Could you check a few things on this model? Use its own coordinates, in mm. A direction names the side the tool comes from. Coordinates: 2 decimals unless noted, no trailing zeros. Loops run counter-clockwise (first coordinate to the right, second up) from the corner with the lowest first, then second, coordinate; pieces in that order, holes last. Notation, with made-up numbers: M 22,-31 L 67,-31 A13 cw 67,-24 Z; hole C -39.5,-26.75 d4. An arc over 180 degrees is marked long. Use one line per item in the form item = value. Start each with the question number.
```python
from build123d import *

# Parameters (mm, degrees)
SKETCH2_R          = 17.5
CUT_EXTRUDE1_DEPTH = 108.121426428
SKETCH3_W          = 10
SKETCH3_H          = 6.6
CUT_EXTRUDE2_DEPTH = 108.121426428
SKETCH4_R          = 4
CUT_EXTRUDE3_DEPTH = 10
CUT_EXTRUDE4_DEPTH = 108.121426428


with BuildPart() as part:
    # Sketch1 → Revolve1 (revolve)
    with BuildSketch(Plane.XY, mode=Mode.PRIVATE) as revolve1_sk:
        with BuildLine():
            Line((-55, 0), (0, 0))
            Line((0, 0), (0, 65))
            Line((0, 65), (-15, 65))
            ThreePointArc((-15, 65), (-18.535533906, 63.535533906), (-20, 60))
            Line((-20, 60), (-20, 38))
            ThreePointArc((-20, 38), (-22.343145751, 32.343145751), (-28, 30))
            Line((-28, 30), (-52, 30))
            ThreePointArc((-52, 30), (-54.121320344, 29.121320344), (-55, 27))
            Line((-55, 27), (-55, 0))
        make_face()
    revolve(revolve1_sk.sketch.rotate(Axis((-55, 0, 0), (1, 0, 0)), 90), axis=Axis((-55, 0, 0), (1, 0, 0)))

    # Sketch2 → Cut-Extrude1 (cut, through all)
    with BuildSketch(Plane.ZY.offset(55)):
        Circle(SKETCH2_R)
    extrude(amount=-CUT_EXTRUDE1_DEPTH, mode=Mode.SUBTRACT)

    # Sketch3 → Cut-Extrude2 (cut, through all)
    with BuildSketch(Plane(origin=(0, 0, 0), x_dir=(0, 0, -1), z_dir=(1, 0, 0))):
        with Locations((0, 17.5)):
            Rectangle(SKETCH3_W, SKETCH3_H)
    extrude(amount=-CUT_EXTRUDE2_DEPTH, mode=Mode.SUBTRACT)

    # Sketch4 → Cut-Extrude3 (cut)
    with BuildSketch(Plane(origin=(0, -30, 0), x_dir=(-1, 0, 0), z_dir=(0, -1, 0))):
        with Locations(Location((40.229772479, 0, 0), (0, 0, 90))):
            Circle(SKETCH4_R)
    extrude(amount=-CUT_EXTRUDE3_DEPTH, mode=Mode.SUBTRACT)

    # Sketch5 → Cut-Extrude4 (cut, through all)
    with BuildSketch(Plane(origin=(0, 0, 0), x_dir=(0, 0, -1), z_dir=(1, 0, 0))):
        with BuildLine():
            ThreePointArc((-48.88940991, 26.321058084), (-49.547284726, 19.781093542), (-45.084090379, 14.955761253))
            ThreePointArc((-45.084090379, 14.955761253), (-41.13620668, 23.75), (-35.494114368, 31.566086948))
            ThreePointArc((-35.494114368, 31.566086948), (-41.904571885, 33.01866049), (-47.23940991, 29.178941916))
            Line((-47.23940991, 29.178941916), (-48.88940991, 26.321058084))
        make_face()
        with BuildLine():
            ThreePointArc((-35.494114368, 31.566086948), (-41.13620668, 23.75), (-45.084090379, 14.955761253))
            ThreePointArc((-45.084090379, 14.955761253), (-39.421242138, 14.734980037), (-35.033003449, 18.321058084))
            Line((-35.033003449, 18.321058084), (-33.383003449, 21.178941916))
            ThreePointArc((-33.383003449, 21.178941916), (-32.471488106, 26.772307122), (-35.494114368, 31.566086948))
        make_face()
        with BuildLine():
            ThreePointArc((35.033003449, 18.321058084), (39.421242138, 14.734980037), (45.084090379, 14.955761253))
            ThreePointArc((45.084090379, 14.955761253), (41.13620668, 23.75), (35.494114368, 31.566086948))
            ThreePointArc((35.494114368, 31.566086948), (32.471488106, 26.772307122), (33.383003449, 21.178941916))
            Line((33.383003449, 21.178941916), (35.033003449, 18.321058084))
        make_face()
        with BuildLine():
            ThreePointArc((35.494114368, 31.566086948), (41.13620668, 23.75), (45.084090379, 14.955761253))
            ThreePointArc((45.084090379, 14.955761253), (49.547284726, 19.781093542), (48.88940991, 26.321058084))
            Line((48.88940991, 26.321058084), (47.23940991, 29.178941916))
            ThreePointArc((47.23940991, 29.178941916), (41.904571885, 33.01866049), (35.494114368, 31.566086948))
        make_face()
        with BuildLine():
            Line((1.65, -39.5), (-1.65, -39.5))
            ThreePointArc((-1.65, -39.5), (-6.949754033, -41.507287159), (-9.589976011, -46.521848202))
            ThreePointArc((-9.589976011, -46.521848202), (0, -47.5), (9.589976011, -46.521848202))
            ThreePointArc((9.589976011, -46.521848202), (6.949754033, -41.507287159), (1.65, -39.5))
        make_face()
        with BuildLine():
            ThreePointArc((9.589976011, -46.521848202), (0, -47.5), (-9.589976011, -46.521848202))
            ThreePointArc((-9.589976011, -46.521848202), (-7.642712841, -52.799754033), (-1.65, -55.5))
            Line((-1.65, -55.5), (1.65, -55.5))
            ThreePointArc((1.65, -55.5), (7.642712841, -52.799754033), (9.589976011, -46.521848202))
        make_face()
    extrude(amount=-CUT_EXTRUDE4_DEPTH, mode=Mode.SUBTRACT)

    # Cut-Extrude5 cone 1 section (on through the dimple's axis) → Cut-Extrude5 (revolve, cut)
    with BuildSketch(Plane(origin=(0, 47.5, 0), x_dir=(0, 0, -1), z_dir=(0, 1, 0))):
        Polygon((0, 0), (7, 0), (0, 93.336682434), align=None)
    revolve(axis=Axis((0, 47.5, 0), (-1, 0, 0)), mode=Mode.SUBTRACT)

    # Cut-Extrude5 cone 2 section (on through the dimple's axis) → Cut-Extrude5 cone 2 (revolve, cut)
    with BuildSketch(Plane(origin=(0, -23.75, -41.13620668), x_dir=(0, 0, -1), z_dir=(0, 1, 0))):
        Polygon((0, 0), (7, 0), (0, 93.336682434), align=None)
    revolve(axis=Axis((0, -23.75, -41.13620668), (-1, 0, 0)), mode=Mode.SUBTRACT)

    # Cut-Extrude5 cone 3 section (on through the dimple's axis) → Cut-Extrude5 cone 3 (revolve, cut)
    with BuildSketch(Plane(origin=(0, -23.75, 41.13620668), x_dir=(0, 0, -1), z_dir=(0, 1, 0))):
        Polygon((0, 0), (7, 0), (0, 93.336682434), align=None)
    revolve(axis=Axis((0, -23.75, 41.13620668), (-1, 0, 0)), mode=Mode.SUBTRACT)


solid = part.part
```
Item 1: I want a section at B-B (x = -32.5). Write out the boundary of the cut face in (y, z), plus the area to 3 significant figures.
Item 2: Please list where these lines run through material, in increasing order: line 1 along Y through (x, z) = (-14, 0); line 2 along X through (y, z) = (-26, 0); line 3 along Y through (x, z) = (-13, 9).
Item 3: I want a section at A-A (y = 0). Write out the boundary of the cut face in (x, z).
Item 4: I want a section at C-C (z = 0). Count the separate pieces of the cut face and the enclosed holes in it, plus the area to 3 significant figures.
Item 5: For faces 1 (the cylindrical face through (-44.135, -25.071, 0.867)), 2 (the flat face through (0, 14, -14)), 3 (the cylindrical face through (-40.168, 29.287, -6.503)), 4 (the conical face through (-10.14, 53.59, 1.35)), 5 (the flat face through (-10, -55.5, 0)), which set-ups out of +Z, -Z, +X, -X, +Y, -Y let a thin tool reach every point of the face, with its end or its side?
Item 6: I'm going to push flat-ended pins straight in: P1, Ø8, axis at x = -21.5, z = 25.5, coming from the +Y side; P2, Ø3.5, axis at x = -11.5, z = 0, coming from the -Y side; P3, Ø2.5, axis at x = -39, z = -2, coming from the -Y side; P4, Ø2, axis at y = 45, z = 46, coming from the +X side. Where does each tip first touch, or does it pass through?
Item 7: Thinking about a two-plate mould opening in Y: for faces 6 (the flat face through (-20, 39, -1)), 7 (the conical face through (-10.1, -25.6, -47.1)), 8 (the flat face through (-40, -20, 0)), which applies, pulls with the +Y half, pulls with the -Y half, needs draft (parallel to the pull), parting line crosses it, or undercut?
Worked answers:
q1.outline = C 0,0 d60; hole M 16.77,-5 L 20.8,-5 L 20.8,5 L 16.77,5 A17.5 ccw long Z
q1.area = 1,830 mm²
q2.line_1 = -65 to -55.5, -39.5 to -17.5, 20.8 to 41.55, 53.45 to 65
q2.line_2 = -55 to -44.23, -36.23 to 0
q2.line_3 = -64.37 to -50.66, -44.34 to -15.01, 15.01 to 64.37
q3.outline = M -55,-27 A3 ccw -52,-30 L -28,-30 A8 cw -20,-38 L -20,-60 A5 ccw -15,-65 L 0,-65 L 0,-17.5 L -55,-17.5 Z; M -55,17.5 L 0,17.5 L 0,65 L -15,65 A5 ccw -20,60 L -20,38 A8 cw -28,30 L -52,30 A3 ccw -55,27 Z
q4.separate_pieces = 4
q4.enclosed_holes = 0
q4.area = 1,960 mm²
q5.face_1 = -Y
q5.face_2 = +Z, -Z, +X, +Y, -Y
q5.face_3 = -X
q5.face_4 = +X
q5.face_5 = +X, -X
q6.P1 = 59.51
q6.P2 = -65
q6.P3 = -20
q6.P4 = 0
q7.face_6 = needs draft
q7.face_7 = undercut
q7.face_8 = pulls with the -Y half
